For this review, use the dimensioned drawing (mm, ordinates from the lowest corner) and the shaded views. A direction names the side the tool comes from. Coordinates: 2 decimals unless noted, no trailing zeros. Loops run counter-clockwise (first coordinate to the right, second up) from the corner with the lowest first, then second, coordinate; pieces in that order, holes last. Notation, with made-up numbers: (35.5, -0.5) - (69.5, -0.5) arc R15 cw to (69.5, 4.5) - close; hole circle Ø5 at (1.25, 64). An arc over 180 degrees is marked (long way). One line per item, written item: value. Start each with the question number.
1. Insertion check: P1, Ø3.5, axis at x = 18.79, z = 61.21, coming from the -Y side; P2, Ø5, axis at x = 40.5, y = 3.5, coming from the -Z side; P3, Ø1.5, axis at x = 41, y = 13, coming from the -Z side. Each pin has a flat end and moves straight along its axis. Give the tip position at first contact, or say it passes through.
2. We need section A-A, the plane z = 40. Give the boundary of the cut face in (x, y), then the cut area to 3 significant figures.
3. We need section B-B, the plane x = 40. Give the boundary of the cut face in (y, z), then the cut area to 3 significant figures.
4. We need section C-C, the plane y = 12. Count the separate pieces of the cut face and the enclosed holes in it, then the cut area to 3 significant figures.
5. For the marked faces 1 and 2, list the 3-axis set-ups (+Z, -Z, +X, -X, +Y, -Y) from which the entire face can be reached by the end or side of a thin tool; tool diameter is ignored.
6. We need section D-D, the plane x = 12.5. Give the boundary of the cut face in (y, z) (1 decimal), then the cut area to 3 significant figures.
7. To check wall thickness, follow line 1 (Z direction, x = 40, y = 12.65); line 2 (Y direction, x = 32, z = 3.5); line 3 (Z direction, x = 40, y = 3.5). State the ranges of each line that lie inside material, in increasing order.
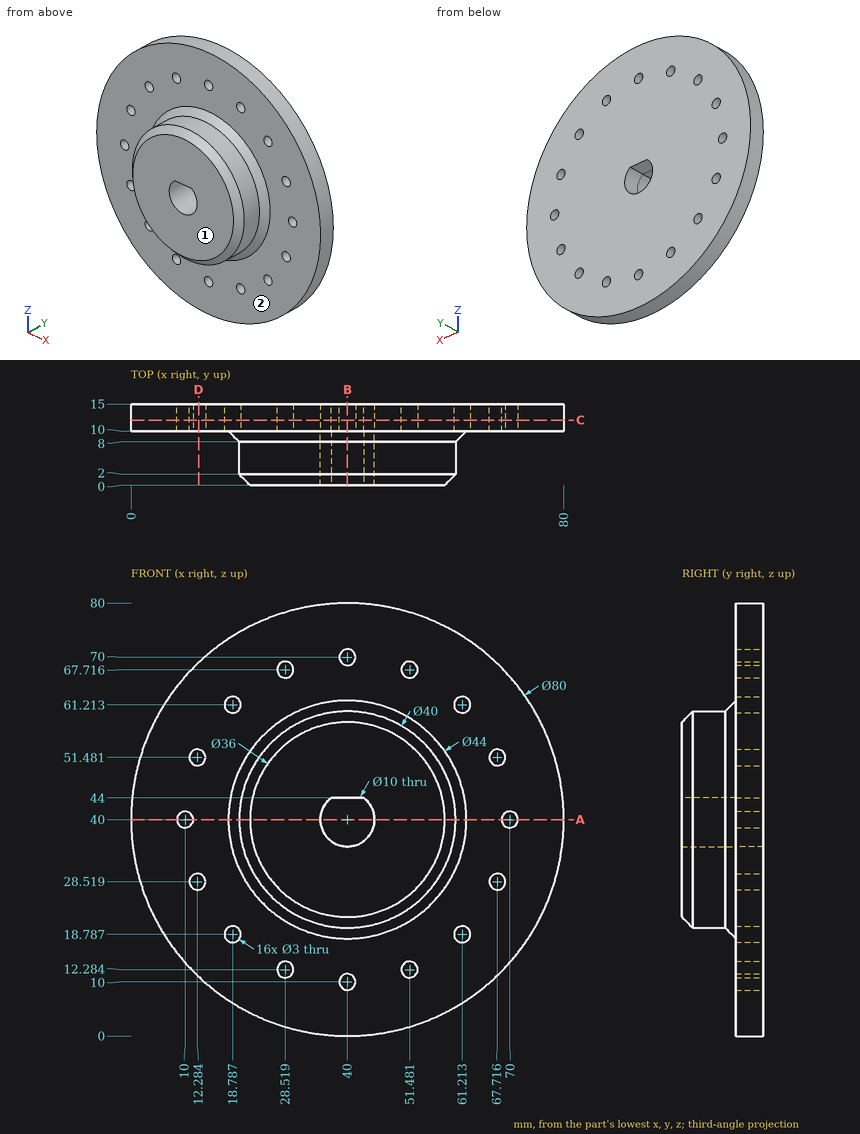
Findings below:
1. P1: y = 10
1. P2: z = 20
1. P3: z = 0
2. outline: (0, 10) - (8.5, 10) - (8.5, 15) - (0, 15) - close; (11.5, 10) - (18, 10) - (20, 8) - (20, 2) - (22, 0) - (35, 0) - (35, 15) - (11.5, 15) - close; (45, 0) - (58, 0) - (60, 2) - (60, 8) - (62, 10) - (68.5, 10) - (68.5, 15) - (45, 15) - close; (71.5, 10) - (80, 10) - (80, 15) - (71.5, 15) - close
2. area: 620 mm2
3. outline: (0, 22) - (2, 20) - (8, 20) - (10, 18) - (10, 11.5) - (15, 11.5) - (15, 35) - (0, 35) - close; (0, 44) - (15, 44) - (15, 68.5) - (10, 68.5) - (10, 62) - (8, 60) - (2, 60) - (0, 58) - close; (10, 0) - (15, 0) - (15, 8.5) - (10, 8.5) - close; (10, 71.5) - (15, 71.5) - (15, 80) - (10, 80) - close
3. area: 635 mm2
4. separate pieces: 1
4. enclosed holes: 17
4. area: 4,840 mm2
5. face 1: +Z, -Z, +X, -X, -Y
5. face 2: -Y
6. outline: (10, 11) - (15, 11) - (15, 27) - (10, 27) - close; (10, 30) - (15, 30) - (15, 50) - (10, 50) - close; (10, 53) - (15, 53) - (15, 69) - (10, 69) - close
6. area: 261 mm2
7. line 1: 0 to 8.5, 11.5 to 35, 44 to 68.5, 71.5 to 80
7. line 2: 10 to 15
7. line 3: 20 to 35, 44 to 60
